from build123d import *

# Parameters (mm, degrees)
SKETCH_1_W                       = 1.5
SKETCH_1_H                       = 500
SM_BASE_FLANGE_1_DEPTH           = 385
SM_EDGE_FLANGE_1_STRIP_W         = 7.4732
SM_EDGE_FLANGE_1_STRIP_H         = 1.5
SM_EDGE_FLANGE_1_STRIP_CUT_DEPTH = 385
SM_EDGE_FLANGE_1_DEPTH           = 385
SKETCH_12_W                      = 16.530990935
SKETCH_12_H                      = 8.400471009
CUT_EXTRUDE_1_DEPTH              = 8
SKETCH_13_R                      = 2.75
CUT_EXTRUDE_2_DEPTH              = 20
SKETCH_14_R                      = 2.75
CUT_EXTRUDE_3_DEPTH              = 10
SKETCH_15_R                      = 2.25
CUT_EXTRUDE_4_DEPTH              = 10


# Sheet-metal steps are written as plain solids
with BuildPart() as part:
    # Sketch 1 → 基体-法兰1 (new body)
    with BuildSketch(Plane.XY):
        with Locations((0.75, 250)):
            Rectangle(SKETCH_1_W, SKETCH_1_H)
    extrude(amount=SM_BASE_FLANGE_1_DEPTH)

    # 边线-法兰1 strip (across the edge) → 边线-法兰1 strip cut (cut)
    with BuildSketch(Plane(origin=(1.5, 500, 0), x_dir=(0, -1, 0), z_dir=(0, 0, 1))):
        with Locations((-1.5, -0.75)):
            Rectangle(SM_EDGE_FLANGE_1_STRIP_W, SM_EDGE_FLANGE_1_STRIP_H)
    extrude(amount=SM_EDGE_FLANGE_1_STRIP_CUT_DEPTH, mode=Mode.SUBTRACT)

    # 边线-法兰1 section (across the edge) → 边线-法兰1 (add)
    with BuildSketch(Plane(origin=(1.5, 500, 0), x_dir=(0, -1, 0), z_dir=(0, 0, 1))):
        with BuildLine():
            Line((0, 0.7366), (0, 13.5))
            Line((0, 13.5), (1.5, 13.5))
            Line((1.5, 13.5), (1.5, 0.7366))
            ThreePointArc((1.5, 0.7366), (1.715745145, 0.215745145), (2.2366, 0))
            Line((2.2366, 0), (2.2366, -1.5))
            ThreePointArc((2.2366, -1.5), (0.655084973, -0.844915027), (0, 0.7366))
        make_face()
    extrude(amount=SM_EDGE_FLANGE_1_DEPTH)

    # 草图12 → 切除-拉伸1 (cut)
    with BuildSketch(Plane.XY.offset(385)):
        with Locations((8.265495468, 501.963635505)):
            Rectangle(SKETCH_12_W, SKETCH_12_H)
    extrude(amount=-CUT_EXTRUDE_1_DEPTH, mode=Mode.SUBTRACT)

    # 草图13 → 切除-拉伸2 (cut)
    with BuildSketch(Plane(origin=(1.5, 0, 0), x_dir=(0, 0, -1), z_dir=(1, 0, 0))):
        with Locations((-288.5, 7.1183)):
            Circle(SKETCH_13_R)
        with Locations((-188.5, 7.1183)):
            Circle(SKETCH_13_R)
        with Locations((-88.5, 7.1183)):
            Circle(SKETCH_13_R)
    extrude(amount=-CUT_EXTRUDE_2_DEPTH, mode=Mode.SUBTRACT)

    # 草图14 → 切除-拉伸3 (cut)
    with BuildSketch(Plane.XZ.offset(-498.5)):
        with Locations(Location((8.6183, 88.5, 0), (0, 0, 270))):
            Circle(SKETCH_14_R)
        with Locations(Location((8.6183, 188.5, 0), (0, 0, 270))):
            Circle(SKETCH_14_R)
        with Locations(Location((8.6183, 288.5, 0), (0, 0, 90))):
            Circle(SKETCH_14_R)
    extrude(amount=-CUT_EXTRUDE_3_DEPTH, mode=Mode.SUBTRACT)

    # 草图15 → 切除-拉伸4 (cut)
    with BuildSketch(Plane.ZY):
        with Locations((382, 98.8817)):
            Circle(SKETCH_15_R)
        with Locations((382, 148.8817)):
            Circle(SKETCH_15_R)
        with Locations((382, 198.8817)):
            Circle(SKETCH_15_R)
        with Locations((382, 298.8817)):
            Circle(SKETCH_15_R)
        with Locations((382, 348.8817)):
            Circle(SKETCH_15_R)
        with Locations((382, 398.8817)):
            Circle(SKETCH_15_R)
    extrude(amount=-CUT_EXTRUDE_4_DEPTH, mode=Mode.SUBTRACT)


solid = part.part
Build history of the part. All positions in model axes, mm. A direction names the side the tool comes from. Coordinates: 2 decimals unless noted, no trailing zeros. Order: outer loops, then holes, each group sorted by start corner. A loop starts at its lowest first (then second) coordinate and runs counter-clockwise, first axis right, second up. Notation, with made-up numbers: M 51.5,1.5 L 59.5,1.5 A5 cw 59.5,8.5 Z; hole C -1,19 d5. An arc over 180 degrees is marked long. One line per question, with ' | ' between items. Start each with the question number.
Q1. Flat gauge pins, fed straight in: pin 1 Ø7 at (y, z) = (298.88, 382) entering from -X; pin 2 Ø2.5 at (y, z) = (98.88, 382) entering from +X; pin 3 Ø1.2 at (x, z) = (0.5, 379.5) entering from +Y; pin 4 Ø7 at (y, z) = (7.12, 288.5) entering from +X. Where does each tip first touch, or does it go through?
Q2. Saw through at B-B (y = 419.5). List the corners of the cut face in (x, z).
Q3. 3-axis set-ups, long thin cutter, end or side, ignore diameter. For faces 1 (the face through (9.95, 500, 185.86)), 2 (the face through (10.1, 498.5, 185.9)): which of +Z, -Z, +X, -X, +Y, -Y reach the whole face in a straight line?
Q4. Saw through at A-A (z = 23). List the corners of the cut face in (x, y), then the cut area to 3 significant figures.
Q5. Probe L1, parallel to Y at x = 13.5, z = 63; L2, parallel to X at y = 208, z = 88; L3, parallel to Y at x = 0.8, z = 288.5. List the from-to ranges inside material, lowest first. Write a range as from..to.
Check values:
1) pin 1: stops at x = 0 | pin 2: passes through | pin 3: stops at y = 497.76 | pin 4: stops at x = 1.5
2) outline: M 0,0 L 1.5,0 L 1.5,385 L 0,385 Z
3) face 1: +Z, -Z, +X, -X, +Y | face 2: +Z, -Z, +X, -Y
4) outline: M 0,0 L 1.5,0 L 1.5,497.76 A0.74 cw 2.24,498.5 L 15,498.5 L 15,500 L 2.24,500 A2.24 ccw 0,497.76 Z | area: 769 mm2
5) L1: y = 498.5..500 | L2: x = 0..1.5 | L3: y = 0..4.37, 9.87..499.48
